```python
from build123d import *

# Parameters (mm, degrees)
BOX009_W          = 20
BOX009_H          = 10
BOX009_DEPTH      = 12
BOX008_W          = 20
BOX008_H          = 12.5
BOX008_DEPTH      = 11
BOX011_W          = 102
BOX011_H          = 113
BOX011_DEPTH      = 21
BOX010_W          = 110
BOX010_H          = 130
BOX010_DEPTH      = 19
CYLINDER001_R     = 3
CYLINDER001_DEPTH = 20
BOX006_W          = 39
BOX006_H          = 17
BOX006_DEPTH      = 10
CYLINDER002_R     = 3
CYLINDER002_DEPTH = 20
BOX005_W          = 39
BOX005_H          = 17
BOX005_DEPTH      = 10
CYLINDER003_R     = 3
CYLINDER003_DEPTH = 20
BOX004_W          = 39
BOX004_H          = 17
BOX004_DEPTH      = 10
CYLINDER005_R     = 3
CYLINDER005_DEPTH = 20
BOX002_W          = 39
BOX002_H          = 17
BOX002_DEPTH      = 10
CYLINDER004_R     = 3
CYLINDER004_DEPTH = 20
BOX003_W          = 39
BOX003_H          = 17
BOX003_DEPTH      = 10
CYLINDER011_R     = 3
CYLINDER011_DEPTH = 20
CYLINDER010_R     = 3
CYLINDER010_DEPTH = 20
CYLINDER009_R     = 3
CYLINDER009_DEPTH = 20
CYLINDER008_R     = 3
CYLINDER008_DEPTH = 20
CYLINDER007_R     = 3
CYLINDER007_DEPTH = 20
CYLINDER006_R     = 3
CYLINDER006_DEPTH = 20
BOX007_W          = 102
BOX007_H          = 54
BOX007_DEPTH      = 10
CYLINDER_R        = 3
CYLINDER_DEPTH    = 20
BOX001_W          = 39
BOX001_H          = 17
BOX001_DEPTH      = 10
BOX_W             = 110
BOX_H             = 130
BOX_DEPTH         = 4
FILLET_R          = 2.5


with BuildPart() as obj1:
    # Box009 → Box009 (new body)
    with BuildSketch(Plane(origin=(62, 112, 3), x_dir=(0, 1, 0), z_dir=(0, 0, 1))):
        with Locations((10, 5)):
            Rectangle(BOX009_W, BOX009_H)
    extrude(amount=BOX009_DEPTH)


with BuildPart() as usbport:
    # Box008 → Box008 (new body)
    with BuildSketch(Plane(origin=(92, 112, 3), x_dir=(0, 1, 0), z_dir=(0, 0, 1))):
        with Locations((10, 6.25)):
            Rectangle(BOX008_W, BOX008_H)
    extrude(amount=BOX008_DEPTH)


with BuildPart() as obj2:
    # Box011 → Box011 (new body)
    with BuildSketch(Plane(origin=(-2, 4, -2), x_dir=(1, 0, 0), z_dir=(0, 0, 1))):
        with Locations((51, 56.5)):
            Rectangle(BOX011_W, BOX011_H)
    extrude(amount=BOX011_DEPTH)


with BuildPart() as obj3:
    # Box010 → Box010 (new body)
    with BuildSketch(Plane(origin=(-2, -5, -2), x_dir=(1, 0, 0), z_dir=(0, 0, 1))):
        with Locations((55, 65)):
            Rectangle(BOX010_W, BOX010_H)
    extrude(amount=BOX010_DEPTH)

    # Cut019: cut obj2
    add(obj2.part, mode=Mode.SUBTRACT)

    # Cut020: cut Usbport
    add(usbport.part, mode=Mode.SUBTRACT)

    # Cut021: cut obj1
    add(obj1.part, mode=Mode.SUBTRACT)


with BuildPart() as zylinder001:
    # Cylinder001 → Cylinder001 (new body)
    with BuildSketch(Plane(origin=(17, 32, 0), x_dir=(1, 0, 0), z_dir=(0, 0, 1))):
        Circle(CYLINDER001_R)
    extrude(amount=CYLINDER001_DEPTH)


with BuildPart() as cut001:
    # Box006 → Box006 (new body)
    with BuildSketch(Plane(origin=(0, 24, 0), x_dir=(1, 0, 0), z_dir=(0, 0, 1))):
        with Locations((19.5, 8.5)):
            Rectangle(BOX006_W, BOX006_H)
    extrude(amount=BOX006_DEPTH)

    # Cut001: cut Zylinder001
    add(zylinder001.part, mode=Mode.SUBTRACT)


with BuildPart() as zylinder002:
    # Cylinder002 → Cylinder002 (new body)
    with BuildSketch(Plane(origin=(17, 50, 0), x_dir=(1, 0, 0), z_dir=(0, 0, 1))):
        Circle(CYLINDER002_R)
    extrude(amount=CYLINDER002_DEPTH)


with BuildPart() as cut002:
    # Box005 → Box005 (new body)
    with BuildSketch(Plane(origin=(0, 42, 0), x_dir=(1, 0, 0), z_dir=(0, 0, 1))):
        with Locations((19.5, 8.5)):
            Rectangle(BOX005_W, BOX005_H)
    extrude(amount=BOX005_DEPTH)

    # Cut002: cut Zylinder002
    add(zylinder002.part, mode=Mode.SUBTRACT)


with BuildPart() as zylinder003:
    # Cylinder003 → Cylinder003 (new body)
    with BuildSketch(Plane(origin=(17, 106, 0), x_dir=(1, 0, 0), z_dir=(0, 0, 1))):
        Circle(CYLINDER003_R)
    extrude(amount=CYLINDER003_DEPTH)


with BuildPart() as cut003:
    # Box004 → Box004 (new body)
    with BuildSketch(Plane(origin=(0, 97, 0), x_dir=(1, 0, 0), z_dir=(0, 0, 1))):
        with Locations((19.5, 8.5)):
            Rectangle(BOX004_W, BOX004_H)
    extrude(amount=BOX004_DEPTH)

    # Cut003: cut Zylinder003
    add(zylinder003.part, mode=Mode.SUBTRACT)


with BuildPart() as zylinder005:
    # Cylinder005 → Cylinder005 (new body)
    with BuildSketch(Plane(origin=(17, 70, 0), x_dir=(1, 0, 0), z_dir=(0, 0, 1))):
        Circle(CYLINDER005_R)
    extrude(amount=CYLINDER005_DEPTH)


with BuildPart() as cut005:
    # Box002 → Box002 (new body)
    with BuildSketch(Plane(origin=(0, 61, 0), x_dir=(1, 0, 0), z_dir=(0, 0, 1))):
        with Locations((19.5, 8.5)):
            Rectangle(BOX002_W, BOX002_H)
    extrude(amount=BOX002_DEPTH)

    # Cut005: cut Zylinder005
    add(zylinder005.part, mode=Mode.SUBTRACT)


with BuildPart() as zylinder004:
    # Cylinder004 → Cylinder004 (new body)
    with BuildSketch(Plane(origin=(17, 88, 0), x_dir=(1, 0, 0), z_dir=(0, 0, 1))):
        Circle(CYLINDER004_R)
    extrude(amount=CYLINDER004_DEPTH)


with BuildPart() as cut004:
    # Box003 → Box003 (new body)
    with BuildSketch(Plane(origin=(0, 79, 0), x_dir=(1, 0, 0), z_dir=(0, 0, 1))):
        with Locations((19.5, 8.5)):
            Rectangle(BOX003_W, BOX003_H)
    extrude(amount=BOX003_DEPTH)

    # Cut004: cut Zylinder004
    add(zylinder004.part, mode=Mode.SUBTRACT)


with BuildPart() as zylinder011:
    # Cylinder011 → Cylinder011 (new body)
    with BuildSketch(Plane(origin=(81, 49, 0), x_dir=(1, 0, 0), z_dir=(0, 0, 1))):
        Circle(CYLINDER011_R)
    extrude(amount=CYLINDER011_DEPTH)


with BuildPart() as zylinder010:
    # Cylinder010 → Cylinder010 (new body)
    with BuildSketch(Plane(origin=(53, 49, 0), x_dir=(1, 0, 0), z_dir=(0, 0, 1))):
        Circle(CYLINDER010_R)
    extrude(amount=CYLINDER010_DEPTH)


with BuildPart() as zylinder009:
    # Cylinder009 → Cylinder009 (new body)
    with BuildSketch(Plane(origin=(47, 19, 0), x_dir=(1, 0, 0), z_dir=(0, 0, 1))):
        Circle(CYLINDER009_R)
    extrude(amount=CYLINDER009_DEPTH)


with BuildPart() as zylinder008:
    # Cylinder008 → Cylinder008 (new body)
    with BuildSketch(Plane(origin=(97, 25, 0), x_dir=(1, 0, 0), z_dir=(0, 0, 1))):
        Circle(CYLINDER008_R)
    extrude(amount=CYLINDER008_DEPTH)


with BuildPart() as zylinder007:
    # Cylinder007 → Cylinder007 (new body)
    with BuildSketch(Plane(origin=(47, 101, 0), x_dir=(1, 0, 0), z_dir=(0, 0, 1))):
        Circle(CYLINDER007_R)
    extrude(amount=CYLINDER007_DEPTH)


with BuildPart() as zylinder006:
    # Cylinder006 → Cylinder006 (new body)
    with BuildSketch(Plane(origin=(97, 100, 0), x_dir=(1, 0, 0), z_dir=(0, 0, 1))):
        Circle(CYLINDER006_R)
    extrude(amount=CYLINDER006_DEPTH)


with BuildPart() as cut011:
    # Box007 → Box007 (new body)
    with BuildSketch(Plane(origin=(45, 115, 0), x_dir=(0, -1, 0), z_dir=(0, 0, 1))):
        with Locations((51, 27)):
            Rectangle(BOX007_W, BOX007_H)
    extrude(amount=BOX007_DEPTH)

    # Cut006: cut Zylinder006
    add(zylinder006.part, mode=Mode.SUBTRACT)

    # Cut007: cut Zylinder007
    add(zylinder007.part, mode=Mode.SUBTRACT)

    # Cut008: cut Zylinder008
    add(zylinder008.part, mode=Mode.SUBTRACT)

    # Cut009: cut Zylinder009
    add(zylinder009.part, mode=Mode.SUBTRACT)

    # Cut010: cut Zylinder010
    add(zylinder010.part, mode=Mode.SUBTRACT)

    # Cut011: cut Zylinder011
    add(zylinder011.part, mode=Mode.SUBTRACT)


with BuildPart() as zylinder:
    # Cylinder → Cylinder (new body)
    with BuildSketch(Plane(origin=(17, 14, 0), x_dir=(1, 0, 0), z_dir=(0, 0, 1))):
        Circle(CYLINDER_R)
    extrude(amount=CYLINDER_DEPTH)


with BuildPart() as cut:
    # Box001 → Box001 (new body)
    with BuildSketch(Plane(origin=(0, 6, 0), x_dir=(1, 0, 0), z_dir=(0, 0, 1))):
        with Locations((19.5, 8.5)):
            Rectangle(BOX001_W, BOX001_H)
    extrude(amount=BOX001_DEPTH)

    # Cut: cut Zylinder
    add(zylinder.part, mode=Mode.SUBTRACT)


with BuildPart() as base001:
    # Box → Box (new body)
    with BuildSketch(Plane(origin=(-2, -5, -2), x_dir=(1, 0, 0), z_dir=(0, 0, 1))):
        with Locations((55, 65)):
            Rectangle(BOX_W, BOX_H)
    extrude(amount=BOX_DEPTH)

    # Cut012: cut Cut
    add(cut.part, mode=Mode.SUBTRACT)

    # Cut013: cut Cut011
    add(cut011.part, mode=Mode.SUBTRACT)

    # Cut014: cut Cut004
    add(cut004.part, mode=Mode.SUBTRACT)

    # Cut015: cut Cut005
    add(cut005.part, mode=Mode.SUBTRACT)

    # Cut016: cut Cut003
    add(cut003.part, mode=Mode.SUBTRACT)

    # Cut017: cut Cut002
    add(cut002.part, mode=Mode.SUBTRACT)

    # Cut018: cut Cut001
    add(cut001.part, mode=Mode.SUBTRACT)

    # Fusion: union obj3
    add(obj3.part)

    # Fillet
    fillet_edges = [base001.edges().sort_by_distance(p)[0] for p in [
        (-2, -5, 9.5),
        (108, -5, 9.5),
        (108, 125, 9.5),
        (-2, 125, 9.5),
    ]]
    fillet(fillet_edges, radius=FILLET_R)


solid = base001.part
```
Model file for the job. Use its own axes, mm. A direction names the side the tool comes from. Coordinates: 2 decimals unless noted, no trailing zeros. Order: outer loops, then holes, each group sorted by start corner. A loop starts at its lowest first (then second) coordinate and runs counter-clockwise, first axis right, second up. Notation, with made-up numbers: (88.5, 47) - (98.5, 47) arc R20 ccw to (98.5, 85) - close; hole circle Ø5 at (18.25, 16). An arc over 180 degrees is marked (long way). Return JSON: item names as keys, results as strings. Group by question number.
1) Saw through at B-B, the plane x = 81. Write the cut outline in (y, z), plus the area to 3 significant figures.
2) Saw through at D-D, the plane x = 47. Write the cut outline in (y, z), plus the area to 3 significant figures.
3) Saw through at C-C, the plane y = 70. Write the cut outline in (x, z), plus the area to 3 significant figures.
4) Tool access for faces 4 (the flat face through (52, 61, -2)), 5 (the flat face through (17, 50, 2)), 6 (the flat face through (19, 53, 0)): list every direction of +Z, -Z, +X, -X, +Y, -Y with a clear straight run to the whole face (end or side of a thin tool).
5) Mould opens along Y. For faces 1 (the flat face through (52, -5, 7)), 2 (the flat face through (19.2, 103.7, 0)), 3 (the flat face through (52, 121, 9)) say: released by +Y, released by -Y, zero draft, split by the parting line, or undercut.
6) Saw through at A-A, the plane z = 7. Write the cut outline in (x, y).
7) Probe line 1 (Y direction, x = 32.5, z = 15.5); line 2 (Y direction, x = 78.5, z = 0.5); line 3 (X direction, y = 9.5, z = 9.75). List the from-to ranges inside material, lowest first. Write a range as from..to.
8) Flat gauge pins, fed straight in: P1, Ø16, axis at x = 72.5, y = 80, coming from the +Z side; P2, Ø6.5, axis at x = 16, y = 89.5, coming from the +Z side; P3, Ø8, axis at y = 15.5, z = 8, coming from the -X side. Where does each tip first touch, or does it go through?
Values found:
{
 "1": {"outline": "(-5, -2) - (125, -2) - (125, 3) - (117, 3) - (117, 2) - (115, 2) - (115, 0) - (52, 0) - (52, 2) - (46, 2) - (46, 0) - (13, 0) - (13, 2) - (4, 2) - (4, 17) - (-5, 17) - close; (117, 14) - (125, 14) - (125, 17) - (117, 17) - close", "area": "495 mm²"},
 "2": {"outline": "(-5, -2) - (125, -2) - (125, 17) - (117, 17) - (117, 2) - (115, 2) - (115, 0) - (104, 0) - (104, 2) - (98, 2) - (98, 0) - (22, 0) - (22, 2) - (16, 2) - (16, 0) - (13, 0) - (13, 2) - (4, 2) - (4, 17) - (-5, 17) - close", "area": "595 mm²"},
 "3": {"outline": "(-2, -2) - (108, -2) - (108, 17) - (100, 17) - (100, 2) - (99, 2) - (99, 0) - (45, 0) - (45, 2) - (39, 2) - (39, 0) - (20, 0) - (20, 2) - (14, 2) - (14, 0) - (0, 0) - (0, 2) - (-2, 2) - close", "area": "386 mm²"},
 "4": {"face 4": "-Z, +X, -X, +Y, -Y", "face 5": "+Z, -X", "face 6": "+Z"},
 "5": {"face 1": "released by -Y", "face 2": "undercut", "face 3": "zero draft"},
 "6": {"outline": "(-2, -2.5) arc R2.5 ccw to (0.5, -5) - (105.5, -5) arc R2.5 ccw to (108, -2.5) - (108, 122.5) arc R2.5 ccw to (105.5, 125) - (92, 125) - (92, 117) - (100, 117) - (100, 4) - (-2, 4) - close; (-2, 117) - (52, 117) - (52, 125) - (0.5, 125) arc R2.5 ccw to (-2, 122.5) - close; (62, 117) - (79.5, 117) - (79.5, 125) - (62, 125) - close"},
 "7": {"line 1": "y = -5..4, 117..125", "line 2": "y = -5..13, 47.34..50.66, 115..125", "line 3": "x = 100..108"},
 "8": {"P1": "stops at z = 0", "P2": "stops at z = 2", "P3": "stops at x = 100"}
}
